Design review of the part built by this model. Coordinates are the model's own, in mm. A direction names the side the tool comes from. Give positions to 0.01 mm unless a question says otherwise; leave off trailing zeros. Loops run counter-clockwise (first coordinate to the right, second up) from the corner with the lowest first, then second, coordinate; pieces in that order, holes last. Notation, with made-up numbers: (56, 47) - (88, 47) arc R29 cw to (88, 76) - close; hole circle Ø5 at (87, 24.25). An arc over 180 degrees is marked (long way). Put each result on its own line as item: value. Start each with the question number.
```python
from build123d import *

# Parameters (mm, degrees)
SKETCH1_R           = 3.81
BOSS_EXTRUDE1_DEPTH = 23.622


with BuildPart() as part:
    # Sketch1 → Boss-Extrude1 (new body)
    with BuildSketch(Plane.XY):
        with Locations((1.524, 0)):
            Circle(SKETCH1_R)
        with BuildLine():
            ThreePointArc((0, -0.762), (-0.762, 0), (0, 0.762))
            Line((0, 0.762), (0.762, 0.762))
            Line((0.762, 0.762), (0.762, 1.524))
            ThreePointArc((0.762, 1.524), (1.524, 2.286), (2.286, 1.524))
            Line((2.286, 1.524), (2.286, 0.762))
            Line((2.286, 0.762), (3.048, 0.762))
            ThreePointArc((3.048, 0.762), (3.81, 0), (3.048, -0.762))
            Line((3.048, -0.762), (2.286, -0.762))
            Line((2.286, -0.762), (2.286, -1.524))
            ThreePointArc((2.286, -1.524), (1.524, -2.286), (0.762, -1.524))
            Line((0.762, -1.524), (0.762, -0.762))
            Line((0.762, -0.762), (0, -0.762))
        make_face(mode=Mode.SUBTRACT)
    extrude(amount=BOSS_EXTRUDE1_DEPTH)


solid = part.part
```
Item 1: Mouldability with a two-part tool opening along X and no side actions: class faces 1 (the flat face through (3, -1, 23.622)), 2 (the cylindrical face through (1.541, -2.286, 11.646)), 3 (the cylindrical face through (3.81, 0.02, 11.65)), 4 (the cylindrical face through (0.7, -3.72, 11.65)) as pulls with the +X half, pulls with the -X half, needs draft (parallel to the pull), parting line crosses it, or undercut.
Item 2: Consider section C-C (x = 1.75). State the section outline as (y, z) points.
Item 3: Consider section D-D (x = 4.75). State the section outline as (y, z) points, plus the area to 3 significant figures.
Item 4: Machinability: for faces 5 (the flat face through (3, -1, 0)), 6 (the cylindrical face through (1.507, 2.286, 11.646)), which of the approach directions +Z, -Z, +X, -X, +Y, -Y give a long, thin tool a straight path to every point of the face, cutting with its end or side? Answer none if there is none.
Item 5: Consider section B-B (y = 0). State the section outline as (x, z) points.
Item 6: Consider section A-A (z = 9.5). State the section outline as (x, y) points.
Item 7: For P1, Ø0.6, axis at x = 2.5, z = 16.5, coming from the -Y side; P2, Ø0.8, axis at y = -1, z = 8, coming from the -X side; P3, Ø0.8, axis at y = 1.5, z = 13.5, coming from the +X side, all flat-tipped, find the tip position at first contact; note any pin that passes through.
Item 8: For L1, parallel to Y at x = 3.5, z = 20.75; L2, parallel to Y at x = 2.75, z = 9.75; L3, parallel to X at y = 0.5, z = 20, list the stretches that pass through material, from the lowest coordinate up. Write a range as from..to.
Geometry says:
1. face 1: needs draft
1. face 2: undercut
1. face 3: undercut
1. face 4: parting line crosses it
2. outline: (-3.8, 0) - (-2.25, 0) - (-2.25, 23.62) - (-3.8, 23.62) - close; (2.25, 0) - (3.8, 0) - (3.8, 23.62) - (2.25, 23.62) - close
3. outline: (-2.03, 0) - (2.03, 0) - (2.03, 23.62) - (-2.03, 23.62) - close
3. area: 95.8 mm2
4. face 5: -Z, +X, -X, +Y, -Y
4. face 6: +Z, -Z
5. outline: (-2.29, 0) - (-0.76, 0) - (-0.76, 23.62) - (-2.29, 23.62) - close; (3.81, 0) - (5.33, 0) - (5.33, 23.62) - (3.81, 23.62) - close
6. outline: circle Ø7.62 at (1.52, 0); hole (0, -0.76) - (0.76, -0.76) - (0.76, -1.52) arc R0.76 ccw to (2.29, -1.52) - (2.29, -0.76) - (3.05, -0.76) arc R0.76 ccw to (3.05, 0.76) - (2.29, 0.76) - (2.29, 1.52) arc R0.76 ccw to (0.76, 1.52) - (0.76, 0.76) - (0, 0.76) arc R0.76 ccw to start
7. P1: stops at y = -3.75
7. P2: stops at x = -2.24
7. P3: stops at x = 5.17
8. L1: y = -3.26..-0.61, 0.61..3.26
8. L2: y = -3.61..-0.76, 0.76..3.61
8. L3: x = -2.25..-0.58, 3.62..5.3
